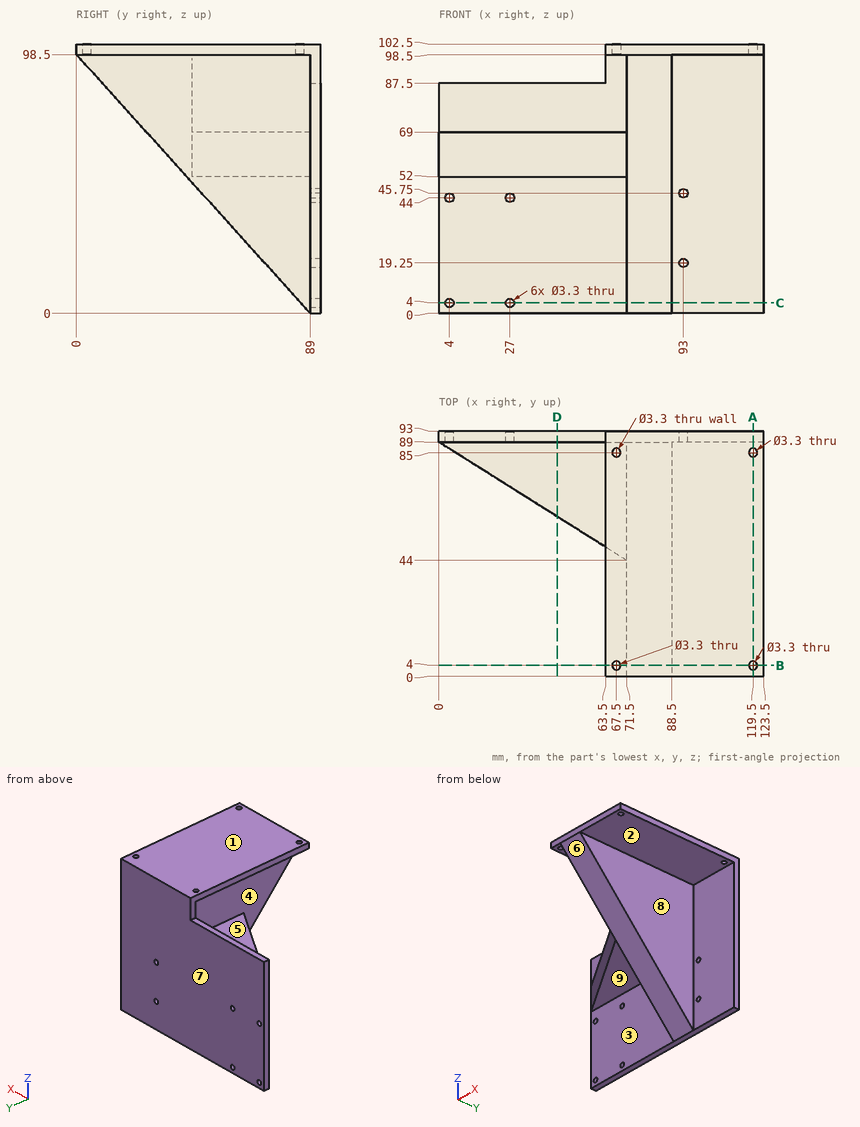
Could you check a few things on this drawing? It's one solid part, dimensions in mm from its lowest x, y, z. A direction names the side the tool comes from. Coordinates: 2 decimals unless noted, no trailing zeros. Order: outer loops, then holes, each group sorted by start corner. A loop starts at its lowest first (then second) coordinate and runs counter-clockwise, first axis right, second up. Notation, with made-up numbers: (88.25, 83.5) - (145.25, 83.5) arc R9 cw to (145.25, 100.5) - close; hole circle Ø9 at (87.5, 88.5). An arc over 180 degrees is marked (long way). Answer as a JSON object with one key per item and string values. Group by question number.
Q1. Imagine slicing it at B-B (y = 4). Please give me the cut outline in (x, z).
Q2. On a 3-axis mill with a long thin cutter (end or side, diameter ignored), from which of +Z, -Z, +X, -X, +Y, -Y can I reach the whole of each face in a straight line? I mean the marked faces 5, 6, 7, 8 and 9. Say none if no direction works.
Q3. Will these pins go through, and if not, where does the flat tip stop? P1, Ø5, axis at x = 54.5, y = 59.5, coming from the +Z side; P2, Ø4.5, axis at y = 64, z = 92.5, coming from the -X side; P3, Ø10, axis at x = 103, y = 31.5, coming from the -Z side; P4, Ø2.5, axis at x = 27, z = 4, coming from the -Y side.
Q4. We'd pull the mould along Z, two halves only. Please class the marked faces 1, 2, 3 and 4: +Z half, -Z half, draft (parallel to the pull), parting line (faces both ways), or undercut.
Q5. Imagine slicing it at C-C (z = 4). Please give me the cut outline in (x, y), and give its area (3 significant figures).
Q6. Imagine slicing it at D-D (x = 45). Please give me the cut outline in (y, z), and give its area (3 significant figures).
Q7. I need wall thicknesses on line 1 (X direction, y = 90, z = 4); line 2 (Y direction, x = 67.5, z = 100.4); line 3 (X direction, y = 85, z = 101.25). Which ranges of each line are inside material? Lowest first, please. Write a range as from..to.
Q8. Imagine slicing it at A-A (x = 119.5). Please give me the cut outline in (y, z).
Determined:
{
 "1": {"outline": "(63.5, 98.5) - (65.85, 98.5) - (65.85, 102.5) - (63.5, 102.5) - close; (69.15, 98.5) - (71.5, 98.5) - (71.5, 94.07) - (88.5, 94.07) - (88.5, 98.5) - (117.85, 98.5) - (117.85, 102.5) - (69.15, 102.5) - close; (121.15, 98.5) - (123.5, 98.5) - (123.5, 102.5) - (121.15, 102.5) - close"},
 "2": {"face 5": "-X, -Y", "face 6": "-Z, +X, -X, -Y", "face 7": "+Z, -Z, +X, -X, +Y", "face 8": "-Z, +X, -Y", "face 9": "-Z, -X, -Y"},
 "3": {"P1": "stops at z = 69", "P2": "stops at x = 71.5", "P3": "stops at z = 98.5", "P4": "passes through"},
 "4": {"face 1": "+Z half", "face 2": "-Z half", "face 3": "draft", "face 4": "undercut"},
 "5": {"outline": "(0, 89) - (2.35, 89) - (2.35, 93) - (0, 93) - close; (5.65, 89) - (25.35, 89) - (25.35, 93) - (5.65, 93) - close; (28.65, 89) - (71.5, 89) - (71.5, 85.39) - (88.5, 85.39) - (88.5, 89) - (123.5, 89) - (123.5, 93) - (28.65, 93) - close", "area": "529 mm2"},
 "6": {"outline": "(60.68, 52) - (89, 52) - (89, 0) - (93, 0) - (93, 87.5) - (89, 87.5) - (89, 69) - (60.68, 69) - close", "area": "831 mm2"},
 "7": {"line 1": "x = 0..2.35, 5.65..25.35, 28.65..123.5", "line 2": "y = 0..2.35, 5.65..83.35, 86.65..93", "line 3": "x = 63.5..65.85, 69.15..117.85, 121.15..123.5"},
 "8": {"outline": "(0, 98.5) - (2.35, 98.5) - (2.35, 102.5) - (0, 102.5) - close; (5.65, 98.5) - (83.35, 98.5) - (83.35, 102.5) - (5.65, 102.5) - close; (86.65, 98.5) - (89, 98.5) - (89, 0) - (93, 0) - (93, 102.5) - (86.65, 102.5) - close"}
}
